Could you check a few things on this drawing? It's one solid part, dimensions in mm from its lowest x, y, z. A direction names the side the tool comes from. Give positions to 0.01 mm unless a question says otherwise; leave off trailing zeros. Loops run counter-clockwise (first coordinate to the right, second up) from the corner with the lowest first, then second, coordinate; pieces in that order, holes last. Notation, with made-up numbers: M 75,83 L 108,83 A7 ccw 108,94 Z; hole C 69.5,-19.5 d5. An arc over 180 degrees is marked long. Write each question's results on one line, items separated by ' | '. Start each with the question number.
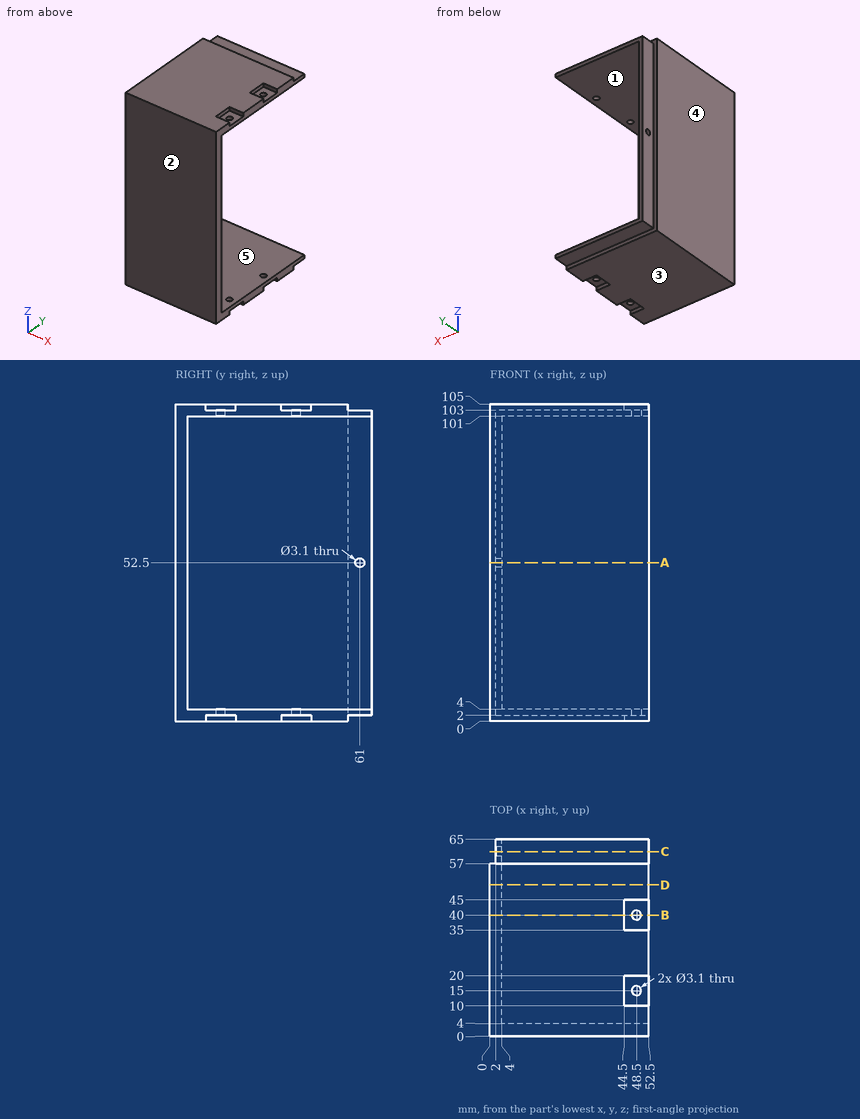
1) If we section it at C-C on y = 61: Write out the boundary of the cut face in (x, z), plus the area to 3 significant figures.
2) Which directions (+Z, -Z, +X, -X, +Y, -Y) give clear straight access to the entire face, cutting with the end or side of a thin tool? Please do the marked faces 1 and 2.
3) If we section it at B-B on y = 40: Write out the boundary of the cut face in (x, z).
4) Please list where these lines run through material, in increasing order: line 1 (Y direction, x = 48.5, z = 102.1); line 2 (Z direction, x = 19, y = 23.5); line 3 (Z direction, x = 47, y = 39.5). Write a range as from..to.
5) Thinking about a two-plate mould opening in Z: for the marked faces 3, 4 and 5, which applies, pulls with the +Z half, pulls with the -Z half, needs draft (parallel to the pull), parting line crosses it, or undercut?
6) If we section it at D-D on y = 50: Write out the boundary of the cut face in (x, z).
7) I'm going to push flat-ended pins straight in: P1, Ø3, axis at x = 13.5, z = 14.5, coming from the +Y side; P2, Ø1.6, axis at y = 16.5, z = 1, coming from the +X side; P3, Ø1, axis at x = 48.5, z = 104, coming from the +Y side; P4, Ø1.9, axis at x = 48.5, y = 15, coming from the -Z side. Where does each tip first touch, or does it pass through?
8) If we section it at A-A on z = 52.5: Write out the boundary of the cut face in (x, y).
Calculated:
1) outline: M 2,2 L 52.5,2 L 52.5,4 L 4,4 L 4,50.95 L 2,50.95 Z; M 2,54.05 L 4,54.05 L 4,101 L 52.5,101 L 52.5,103 L 2,103 Z | area: 390 mm2
2) face 1: +X, +Y | face 2: +Z, -Z, +X, -X, -Y
3) outline: M 0,0 L 44.5,0 L 44.5,2 L 46.95,2 L 46.95,4 L 4,4 L 4,101 L 46.95,101 L 46.95,103 L 44.5,103 L 44.5,105 L 0,105 Z; M 50.05,2 L 52.5,2 L 52.5,4 L 50.05,4 Z; M 50.05,101 L 52.5,101 L 52.5,103 L 50.05,103 Z
4) line 1: y = 0..13.45, 16.55..38.45, 41.55..65 | line 2: z = 0..4, 101..105 | line 3: z = 2..4, 101..103
5) face 3: pulls with the -Z half | face 4: needs draft | face 5: undercut
6) outline: M 0,0 L 52.5,0 L 52.5,4 L 4,4 L 4,101 L 52.5,101 L 52.5,105 L 0,105 Z
7) P1: stops at y = 4 | P2: stops at x = 44.5 | P3: stops at y = 57 | P4: passes through
8) outline: M 0,0 L 52.5,0 L 52.5,4 L 4,4 L 4,59.45 L 2,59.45 L 2,57 L 0,57 Z; M 2,62.55 L 4,62.55 L 4,65 L 2,65 Z
